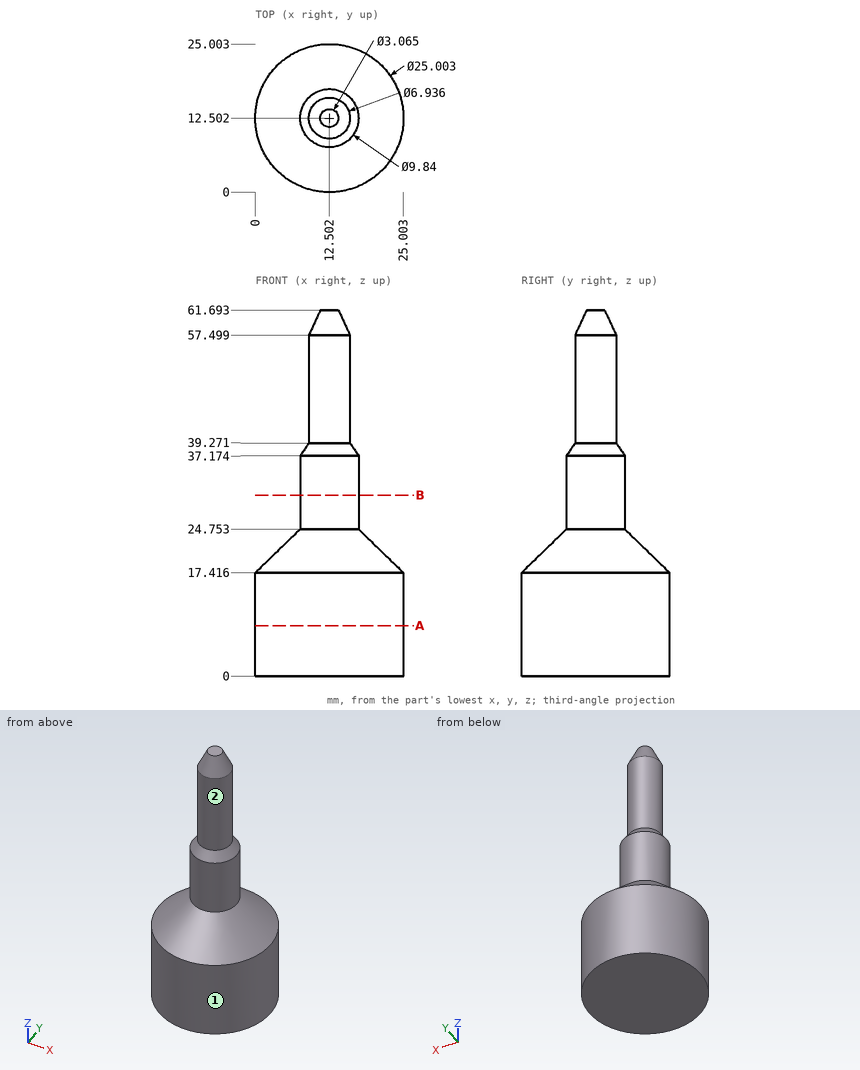
Design review of the part shown in the three views and the two pictorial views. Dimensions are in mm from the part's minimum x, y and z. A direction names the side the tool comes from. Round coordinates to 2 decimals unless told otherwise and drop trailing zeros. Order: outer loops, then holes, each group sorted by start corner. A loop starts at its lowest first (then second) coordinate and runs counter-clockwise, first axis right, second up. Notation, with made-up numbers: (-40, 48.5) - (-25, 48.5) arc R23 cw to (-25, 82.5) - close; hole circle Ø3 at (46, -24). An arc over 180 degrees is marked (long way). One line per question, with ' | ' between items.
Item 1: Wall thickness on line 1 (Z direction, x = 15, y = 12.75) (1 decimal); line 2 (Y direction, x = 15, z = 29.5) (1 decimal); line 3 (X direction, y = 4.75, z = 7) (1 decimal): over which ranges is each line inside the solid? List them lowest first. Write a range as [from, to].
Checks:
line 1: [0, 59.6] | line 2: [8.3, 16.7] | line 3: [2.7, 22.3]
Item 2: Machinability: for the marked faces 1 and 2, which of the approach directions +Z, -Z, +X, -X, +Y, -Y give a long, thin tool a straight path to every point of the face, cutting with its end or side? Answer none if there is none.
Checks:
face 1: +Z, -Z | face 2: +Z
Item 3: Take a section at B-B, the plane z = 30.5. Write out the cut boundary in (x, y).
Checks:
outline: circle Ø9.84 at (12.5, 12.5)
Item 4: Take a section at A-A, the plane z = 8.5. Write out the cut boundary in (x, y), then the cut area to 3 significant figures.
Checks:
outline: circle Ø25 at (12.5, 12.5) | area: 491 mm²
Item 5: For P1, Ø4, axis at y = 17, z = 55, coming from the -X side (1 decimal); P2, Ø10, axis at y = 16, z = 53, coming from the +X side; P3, Ø2, axis at x = 12, z = 25.5, coming from the -Y side, all flat-tipped, find the tip position at first contact; note any pin that passes through.
Checks:
P1: x = 10.1 | P2: x = 15.97 | P3: y = 7.34
